Part model, mm, in its own coordinate system. Coordinates: 2 decimals unless noted, no trailing zeros. Loops run counter-clockwise (first coordinate to the right, second up) from the corner with the lowest first, then second, coordinate; pieces in that order, holes last.
```python
from build123d import *

# Parameters (mm, degrees)
SKETCH1_W           = 16
SKETCH1_H           = 123
BOSS_EXTRUDE1_DEPTH = 1.5
SKETCH2_R           = 1.75
CUT_EXTRUDE1_DEPTH  = 2.5
LPATTERN1_COUNT     = 3
LPATTERN1_PITCH     = 47.5


with BuildPart() as part:
    # Sketch1 → Boss-Extrude1 (new body)
    with BuildSketch(Plane.XY):
        with Locations((8, 61.5)):
            Rectangle(SKETCH1_W, SKETCH1_H)
    extrude(amount=BOSS_EXTRUDE1_DEPTH)

    # Sketch2 → Cut-Extrude1 (cut, through all)
    with BuildSketch(Plane.XY.offset(1.5)):
        with Locations((5, 20)):
            Circle(SKETCH2_R)
    cut_extrude1 = extrude(amount=-CUT_EXTRUDE1_DEPTH, mode=Mode.SUBTRACT)

    # LPattern1: Cut-Extrude1 ×3
    with Locations(*[(0, i * LPATTERN1_PITCH, 0) for i in range(1, LPATTERN1_COUNT)]):
        add(cut_extrude1, mode=Mode.SUBTRACT)


solid = part.part
```
Q1. Mould opens along Y. For faces 1 (the cylindrical face through (3.61, 66.44, 0.76)), 2 (the flat face through (8, 62, 1.5)) say: released by +Y, released by -Y, zero draft, split by the parting line, or undercut.
Q2. Saw through at B-B (x = 5). List the corners of the cut face in (y, z), plus the area to 3 significant figures.
Q3. Probe line 1 (Y direction, x = 5, z = 0.5); line 2 (Y direction, x = 6.5, z = 0.1); line 3 (X direction, y = 66, z = 1.35). List the from-to ranges inside material, lowest first.
Q4. Saw through at A-A (y = 20). List the corners of the cut face in (x, z), plus the area to 4 significant figures.
Checked values:
1. face 1: undercut
1. face 2: zero draft
2. outline: (0, 0) - (18.25, 0) - (18.25, 1.5) - (0, 1.5) - close; (21.75, 0) - (65.75, 0) - (65.75, 1.5) - (21.75, 1.5) - close; (69.25, 0) - (113.25, 0) - (113.25, 1.5) - (69.25, 1.5) - close; (116.75, 0) - (123, 0) - (123, 1.5) - (116.75, 1.5) - close
2. area: 169 mm2
3. line 1: y = 0 to 18.25, 21.75 to 65.75, 69.25 to 113.25, 116.75 to 123
3. line 2: y = 0 to 19.1, 20.9 to 66.6, 68.4 to 114.1, 115.9 to 123
3. line 3: x = 0 to 4.1, 5.9 to 16
4. outline: (0, 0) - (3.25, 0) - (3.25, 1.5) - (0, 1.5) - close; (6.75, 0) - (16, 0) - (16, 1.5) - (6.75, 1.5) - close
4. area: 18.75 mm2
